Part model, mm, in its own coordinate system. Face numbers are marked on the shaded views. Coordinates: 2 decimals unless noted, no trailing zeros. Loops run counter-clockwise (first coordinate to the right, second up) from the corner with the lowest first, then second, coordinate; pieces in that order, holes last. Notation, with made-up numbers: M -0.5,27.5 L 12.5,27.5 A15 cw 12.5,54.5 Z; hole C -3.5,83.25 d9. An arc over 180 degrees is marked long. Use a Markdown table: item, result. Add a question column.
1) Wall check: probe 1 along Z at (x, y) = (0, -1.8); probe 2 along X at (y, z) = (-6.75, 2); probe 3 along X at (y, z) = (-2.5, 3). Give the ranges that are in metal, low to high. Write a range as from..to.
2) Band-saw the part on C-C (y = -1.5). List the corners of the cut face in (x, z), plus the area to 3 significant figures.
3) Pull direction Z, two halves, no side cores. Call the marked faces 1, 2 and 3: released by +Z, released by -Z, zero draft, split by the parting line, or undercut.
4) Pin check, flat tips, straight feed: pin 1 Ø3 at (y, z) = (-4, -5.5) entering from +X; pin 2 Ø10 at (x, z) = (-4.5, 5.5) entering from +Y; pin 3 Ø3 at (x, y) = (-3, -4.5) entering from -Z; pin 4 Ø1.5 at (x, y) = (4, -6.5) entering from +Z. Stop position of each tip, or through.
from build123d import *

# Parameters (mm, degrees)
F0_R     = 8.5
F0_R_2   = 3.5
F1_DEPTH = 8
F2_R     = 2.5
F3_R     = 2.49999


# Not quite as in the source:
# - a fillet or chamfer is up to 0.001 mm smaller than in the source, because OpenCascade refuses the exact size


with BuildPart() as f1:
    # F0 (on Front) → F1 (new body)
    with BuildSketch(Plane.XZ):
        Circle(F0_R)
        Circle(F0_R_2, mode=Mode.SUBTRACT)
    extrude(amount=F1_DEPTH)

    # F2
    f2_edges = [f1.edges().sort_by_distance(p)[0] for p in [
        (-8.5, -8, 0),
    ]]
    fillet(f2_edges, radius=F2_R)

    # F3 (radius 2.5 in the source; OpenCascade refuses exactly that, so slightly less here)
    f3_edges = [f1.edges().sort_by_distance(p)[0] for p in [
        (-3.5, -8, 0),
    ]]
    fillet(f3_edges, radius=F3_R)


solid = f1.part
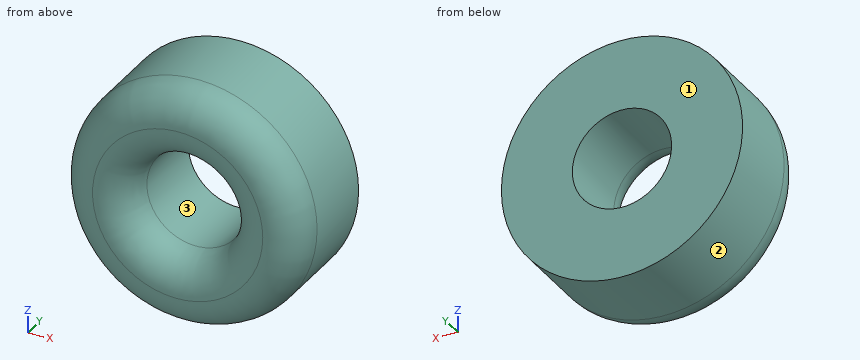
Entries:
| question | item | result |
|---|---|---|
| 1 | probe 1 | -8.5..-3.5, 3.5..8.5 |
| 1 | probe 2 | -7.92..-3.27, 3.27..7.92 |
| 1 | probe 3 | -7.95..-1.8, 1.8..7.95 |
| 2 | outline | C 0,0 d17; hole C 0,0 d7 |
| 2 | area | 188 mm2 |
| 3 | face 1 | zero draft |
| 3 | face 2 | split by the parting line |
| 3 | face 3 | undercut |
| 4 | pin 1 | x = 7.5 |
| 4 | pin 2 | y = 0 |
| 4 | pin 3 | z = -8.37 |
| 4 | pin 4 | z = 7.73 |
